Autodesk Inventor part; units mm, degrees
ref_plane "YZ Plane" through (0, 0, 0) normal (1, 0, 0) x (0, 1, 0)
ref_plane "XZ Plane" through (0, 0, 0) normal (0, 1, 0) x (-1, 0, 0)
ref_plane "XY Plane" through (0, 0, 0) normal (0, 0, 1) x (1, 0, 0)
sketch "Sketch1" plane through (0, 0, 0) normal (0, 0, 1) x (1, 0, 0)
  line L0 (0, 0) -> (260, 0)
  line L1 (260, 0) -> (260, 125)
  line L2 (220, 147) -> (0, 147)
  line L3 (0, 147) -> (0, 0)
  circle A0 centre (240, 135) radius 8
  circle A1 centre (240, 135) radius 10
  line L4 (250, 135) -> (250.202, 135)
  line L5 (230, 135) -> (230, 137)
  arc A2 (230, 137) -> (220, 147) centre (220, 137) ccw
  line L6 (260, 147) -> (260, 147)
  line L7 (250, 135) -> (250, 137)
  line L8 (240, 125) -> (260, 125)
  line L9 (0, 73.5) -> (260, 73.5)
  line L10 (130, 112.7628) -> (117.7684, 112.7628)
  line L11 (99.8322, 119.3312) -> (99.8322, 90.3139)
  line L12 (99.8322, 90.3139) -> (148.259, 90.3139)
  line L13 (148.259, 90.3139) -> (148.259, 44.839)
  line L14 (148.259, 44.839) -> (117.7684, 44.839)
  line L15 (99.8322, 44.839) -> (99.8322, 25.7829)
  line L16 (99.8322, 25.7829) -> (130, 25.7829)
  line L17 (99.8322, 119.3312) -> (99.8322, 127)
  line L18 (99.8322, 127) -> (117.7684, 127)
  line L19 (117.7684, 127) -> (117.7684, 112.7628)
  line L20 (99.8322, 44.839) -> (99.8322, 55.475)
  line L21 (99.8322, 55.475) -> (117.7684, 55.475)
  line L22 (117.7684, 55.475) -> (117.7684, 44.839)
  line L23 (130, 147) -> (130, 112.7628)
  line L24 (130, 25.7829) -> (130, 0)
  line L25 (60, 107) -> (200, 107)
  line L26 (200, 107) -> (200, 40)
  line L27 (200, 40) -> (60, 40)
  line L28 (60, 40) -> (60, 107)
  circle A3 centre (60, 107) radius 1.5
  circle A4 centre (200, 107) radius 1.5
  circle A5 centre (200, 40) radius 1.5
  circle A6 centre (60, 40) radius 1.5
  circle A7 centre (130, 107) radius 1.5
  circle A8 centre (130, 40) radius 1.5
  line L29 (260, 125) -> (265, 125)
  line L30 (265, 125) -> (265, 0)
  line L31 (265, 0) -> (260, 0)
  line L32 (260, 0) -> (260, 125)
  line L33 (265, 0) -> (263, 0)
  line L34 (263, 0) -> (263, 125)
  point P0 (260, 67.5)
  point P1 (200, 73.5)
  point P2 (148.259, 73.5)
  point P3 (99.8322, 107)
  point P4 (128.5, 107)
  point P5 (131.5, 107)
  point P6 (198.5, 107)
  point P7 (200, 105.5)
  dimension "d2" = 16
  dimension "d3" = 20
  dimension "d4" = 135
  dimension "d5" = 2
  dimension "d6" = 260
  dimension "d7" = 147
  dimension "d8" = 10
  dimension "d11" = 22
  dimension "d16" = 40
  dimension "d17" = 40
  dimension "d18" = 60
  dimension "d19" = 60
  dimension "d20" = 3
  dimension "d21" = 3
  dimension "d22" = 3
  dimension "d23" = 3
  dimension "d24" = 140
  dimension "d25" = 67
  dimension "d26" = 3
  dimension "d27" = 3
  dimension "d28" = 70
  dimension "d29" = 70
  dimension "d30" = 5
  dimension "d31" = 2
extrude "Extrusion1" add sketch "Sketch1" along normal blind 2 contours L24 L16 L15 L27 A8 A5 L26 L9 L1 L0 | L1 L29 L34 L31 | L9 L26 A4 L25 A7 L11 L17 L18 L19 L10 L23 L2 A2 L5 A1 L8 L1 | L34 L29 L30 L31 | L13 L12 L11 L25 A7 A4 L26 L9 | L9 L26 A5 L27 A8 L15 L20 L21 L22 L14 L13
sketch "Sketch2" plane through (0, 0, 0) normal (0, 0, -1) x (-1, 0, 0)
  line L0 (-265, 125) -> (-240, 125)
  line L1 (-130, 0) -> (-265, 0)
  line L2 (-265, 125) -> (-263, 125)
  line L3 (-263, 125) -> (-263, 0)
  line L4 (-263, 0) -> (-265, 0)
  line L5 (-265, 0) -> (-265, 125)
  point P0 (0, 0)
  dimension "d32" = 2
extrude "Extrusion2" add sketch "Sketch2" along normal blind 10
sketch "Sketch3" plane through (265, 0, 2) normal (1, 0, 0) x (0, 0, -1)
  line L0 (12, 125) -> (0, 125)
  line L1 (6, 125) -> (6, 0)
  line L2 (12, 0) -> (0, 0)
  circle A0 centre (6, 105) radius 1.5
  circle A1 centre (6, 20) radius 1.5
  point P0 (2, 0)
  dimension "d35" = 3
  dimension "d36" = 3
  dimension "d37" = 20
  dimension "d38" = 20
extrude "Extrusion3" cut sketch "Sketch3" against normal blind 10
properties part number "Coffee_Machine_Base"
CAD build for the part. Positions are in the model's coordinates, mm. A direction names the side the tool comes from. Coordinates: 2 decimals unless noted, no trailing zeros. Write each loop counter-clockwise with the first axis right and the second up, starting at its lowest first coordinate (ties: lowest second). Pieces come first, ordered by that corner, then holes. Notation, with made-up numbers: (58.5, 43) - (110.5, 43) arc R13 ccw to (110.5, 53) - close; hole circle Ø7 at (-24.5, 29.25). An arc over 180 degrees is marked (long way). Use a Markdown table: item, result. Add a question column.
Item 1: Mould opens along X. For faces 3 (the face through (233.01, 127.85, 0.99)), 4 (the face through (198, 75, 0)), 5 (the face through (263, 63, -5)) say: pulls with the +X half, pulls with the -X half, needs draft (parallel to the pull), parting line crosses it, or undercut.
Item 2: Band-saw the part on B-B, the plane x = 249.5. Give the cut face in (y, z).
Item 3: 3-axis set-ups, long thin cutter, end or side, ignore diameter. For faces 1 (the face through (256.3, 125, 0.5)), 2 (the face through (197, 0, 1)): which of +Z, -Z, +X, -X, +Y, -Y reach the whole face in a straight line?
Item 4: Band-saw the part on C-C, the plane x = 184. Give the cut face in (y, z), and give its area (3 significant figures).
Item 5: Band-saw the part on A-A, the plane y = 73. Give the cut face in (x, z), and give its area (3 significant figures).
Item 6: Flat gauge pins, fed straight in: pin 1 (1 mm diameter, centred on x = 117.5, z = 1.5, fed in from -Y); pin 2 (2 mm diameter, centred on y = 57, z = 0.5, fed in from -X); pin 3 (8 mm diameter, centred on x = 177.5, y = 83, fed in from -Z). Where does each tip first touch, or does it go through?
Item 7: Drill centre lines: L1, parallel to Y at x = 200, z = 0.5; L2, parallel to X at y = 107, z = 1.3; L3, parallel to Z at x = 263.65, y = 105. Where is each one in solid material? Low to high. Write a range as from..to.
Numbers:
| question | item | result |
|---|---|---|
| 1 | face 3 | pulls with the +X half |
| 1 | face 4 | needs draft |
| 1 | face 5 | pulls with the -X half |
| 2 | outline | (0, 0) - (125, 0) - (125, 2) - (0, 2) - close |
| 3 | face 1 | +Z, -Z, +X, +Y |
| 3 | face 2 | +Z, -Z, +X, -X, -Y |
| 4 | outline | (0, 0) - (147, 0) - (147, 2) - (0, 2) - close |
| 4 | area | 294 mm2 |
| 5 | outline | (148.26, 0) - (263, 0) - (263, -10) - (265, -10) - (265, 2) - (148.26, 2) - close |
| 5 | area | 253 mm2 |
| 6 | pin 1 | y = 25.78 |
| 6 | pin 2 | x = 148.26 |
| 6 | pin 3 | z = 0 |
| 7 | L1 | 0..38.5, 41.5..105.5, 108.5..147 |
| 7 | L2 | 99.83..128.5, 131.5..198.5, 201.5..265 |
| 7 | L3 | -10..-5.5, -2.5..2 |
